Read the model definition and answer for the solid it produces. Units are mm, in the model's axes. Round coordinates to 2 decimals unless told otherwise and drop trailing zeros. Write each loop counter-clockwise with the first axis right and the second up, starting at its lowest first coordinate (ties: lowest second). Pieces come first, ordered by that corner, then holes. Notation, with made-up numbers: (54, 11.25) - (89, 11.25) arc R20 ccw to (89, 36.25) - close; hole circle Ø1 at (-3, -37.75). An arc over 180 degrees is marked (long way). Use one line per item in the form item = value. Start each with the question number.
1) The part is cut by section A-A, the plane x = 13. Give the vertices of the cut face in (y, z).
2) The part is cut by section C-C, the plane z = 0.85. Count the separate pieces of the cut face and the enclosed holes in it, plus the area to 3 significant figures.
3) The part is cut by section D-D, the plane x = 75. Give the vertices of the cut face in (y, z).
4) Consider line 1 along Y through (x, z) = (29, 2.7); line 2 along Y through (x, z) = (90, 0.4); line 3 along Y through (x, z) = (87, 1.4). Determine where each line is inside the solid, lowest interval first. Write a range as from..to.
5) The part is cut by section B-B, the plane y = 35.5. Give the vertices of the cut face in (x, z), plus the area to 3 significant figures.
from build123d import *

# Parameters (mm, degrees)
ESQUISSE1_W             = 150
ESQUISSE1_H             = 100
BOSS_EXTRU_1_DEPTH      = 3
ESQUISSE3_W             = 130
ESQUISSE3_H             = 10
ENL_V_MAT_EXTRU_1_DEPTH = 3
ESQUISSE12_W            = 10
ESQUISSE12_H            = 3
ENL_V_MAT_EXTRU_3_DEPTH = 10
ESQUISSE13_W            = 15
ESQUISSE13_H            = 14
ENL_V_MAT_EXTRU_4_DEPTH = 10


with BuildPart() as part:
    # Esquisse1 → Boss.-Extru.1 (new body)
    with BuildSketch(Plane.XY):
        with Locations((75, 50)):
            Rectangle(ESQUISSE1_W, ESQUISSE1_H)
    extrude(amount=BOSS_EXTRU_1_DEPTH)

    # Esquisse3 → Enlèv. mat.-Extru.1 (cut)
    with BuildSketch(Plane.XY.offset(3)):
        with Locations((75, 95)):
            Rectangle(ESQUISSE3_W, ESQUISSE3_H)
    extrude(amount=-ENL_V_MAT_EXTRU_1_DEPTH, mode=Mode.SUBTRACT)

    # Esquisse12 → Enlèv. mat.-Extru.3 (cut)
    with BuildSketch(Plane.XY.offset(3)):
        with Locations((12.5, 6.5)):
            Rectangle(ESQUISSE12_W, ESQUISSE12_H)
        with Locations((37.5, 6.5)):
            Rectangle(ESQUISSE12_W, ESQUISSE12_H)
        with Locations((62.5, 6.5)):
            Rectangle(ESQUISSE12_W, ESQUISSE12_H)
        with Locations((87.5, 6.5)):
            Rectangle(ESQUISSE12_W, ESQUISSE12_H)
        with Locations((112.5, 6.5)):
            Rectangle(ESQUISSE12_W, ESQUISSE12_H)
        with Locations((137.5, 6.5)):
            Rectangle(ESQUISSE12_W, ESQUISSE12_H)
    extrude(amount=-ENL_V_MAT_EXTRU_3_DEPTH, mode=Mode.SUBTRACT)

    # Esquisse13 → Enlèv. mat.-Extru.4 (cut)
    with BuildSketch(Plane.XY.offset(3)):
        with Locations((35.259475166, 75.358514873)):
            Rectangle(ESQUISSE13_W, ESQUISSE13_H)
        with Locations((15.259475166, 75.358514873)):
            Rectangle(ESQUISSE13_W, ESQUISSE13_H)
        with Locations((55.259475166, 75.358514873)):
            Rectangle(ESQUISSE13_W, ESQUISSE13_H)
        with Locations((95.259475166, 75.358514873)):
            Rectangle(ESQUISSE13_W, ESQUISSE13_H)
        with Locations((115.259475166, 75.358514873)):
            Rectangle(ESQUISSE13_W, ESQUISSE13_H)
        with Locations((135.259475166, 75.358514873)):
            Rectangle(ESQUISSE13_W, ESQUISSE13_H)
        with Locations((15.259475166, 55.358514873)):
            Rectangle(ESQUISSE13_W, ESQUISSE13_H)
        with Locations((35.259475166, 55.358514873)):
            Rectangle(ESQUISSE13_W, ESQUISSE13_H)
        with Locations((55.259475166, 55.358514873)):
            Rectangle(ESQUISSE13_W, ESQUISSE13_H)
        with Locations((95.259475166, 55.358514873)):
            Rectangle(ESQUISSE13_W, ESQUISSE13_H)
        with Locations((115.259475166, 55.358514873)):
            Rectangle(ESQUISSE13_W, ESQUISSE13_H)
        with Locations((135.259475166, 55.358514873)):
            Rectangle(ESQUISSE13_W, ESQUISSE13_H)
        with Locations((15.259475166, 35.358514873)):
            Rectangle(ESQUISSE13_W, ESQUISSE13_H)
        with Locations((35.259475166, 35.358514873)):
            Rectangle(ESQUISSE13_W, ESQUISSE13_H)
        with Locations((55.259475166, 35.358514873)):
            Rectangle(ESQUISSE13_W, ESQUISSE13_H)
        with Locations((95.259475166, 35.358514873)):
            Rectangle(ESQUISSE13_W, ESQUISSE13_H)
        with Locations((115.259475166, 35.358514873)):
            Rectangle(ESQUISSE13_W, ESQUISSE13_H)
        with Locations((135.259475166, 35.358514873)):
            Rectangle(ESQUISSE13_W, ESQUISSE13_H)
    extrude(amount=-ENL_V_MAT_EXTRU_4_DEPTH, mode=Mode.SUBTRACT)


solid = part.part
Geometry results:
q1.outline = (0, 0) - (5, 0) - (5, 3) - (0, 3) - close; (8, 0) - (28.36, 0) - (28.36, 3) - (8, 3) - close; (42.36, 0) - (48.36, 0) - (48.36, 3) - (42.36, 3) - close; (62.36, 0) - (68.36, 0) - (68.36, 3) - (62.36, 3) - close; (82.36, 0) - (90, 0) - (90, 3) - (82.36, 3) - close
q2.separate_pieces = 1
q2.enclosed_holes = 24
q2.area = 9,740 mm2
q3.outline = (0, 0) - (90, 0) - (90, 3) - (0, 3) - close
q4.line_1 = 0..28.36, 42.36..48.36, 62.36..68.36, 82.36..90
q4.line_2 = 0..5, 8..28.36, 42.36..48.36, 62.36..68.36, 82.36..90
q4.line_3 = 0..5, 8..90
q5.outline = (0, 0) - (7.76, 0) - (7.76, 3) - (0, 3) - close; (22.76, 0) - (27.76, 0) - (27.76, 3) - (22.76, 3) - close; (42.76, 0) - (47.76, 0) - (47.76, 3) - (42.76, 3) - close; (62.76, 0) - (87.76, 0) - (87.76, 3) - (62.76, 3) - close; (102.76, 0) - (107.76, 0) - (107.76, 3) - (102.76, 3) - close; (122.76, 0) - (127.76, 0) - (127.76, 3) - (122.76, 3) - close; (142.76, 0) - (150, 0) - (150, 3) - (142.76, 3) - close
q5.area = 180 mm2
